Work out the finished part from the listing and answer in its coordinate system (mm). A direction names the side the tool comes from. Give positions to 0.01 mm unless a question says otherwise; leave off trailing zeros. Order: outer loops, then holes, each group sorted by start corner. A loop starts at its lowest first (then second) coordinate and runs counter-clockwise, first axis right, second up.
```python
from build123d import *

# Parameters (mm, degrees)
CYLINDER051_R       = 1.8
CYLINDER051_DEPTH   = 20
ARRAY001022_X_COUNT = 2
ARRAY001022_X_PITCH = 42
BOX022_W            = 122
BOX022_H            = 23
BOX022_DEPTH        = 1.4
BOX020_W            = 52
BOX020_H            = 22
BOX020_DEPTH        = 20
BOX019_W            = 62
BOX019_H            = 32
BOX019_DEPTH        = 5.2
FILLET010_R         = 0.7


with BuildPart() as obj1:
    # Cylinder051 → Cylinder051 (new body)
    with BuildSketch(Plane(origin=(10, 27, -5), x_dir=(1, 0, 0), z_dir=(0, 0, 1))):
        Circle(CYLINDER051_R)
    extrude(amount=CYLINDER051_DEPTH)

    # Array001022 X: obj1 ×2


with BuildPart() as obj1_1:
    add(obj1.part)
    with Locations(*[(i * ARRAY001022_X_PITCH, 0, 0) for i in range(1, ARRAY001022_X_COUNT)]):
        add(obj1.part)


with BuildPart() as obj2:
    # Box022 → Box022 (new body)
    with BuildSketch(Plane(origin=(-25, 0, 2), x_dir=(1, 0, 0), z_dir=(0, 0, 1))):
        with Locations((61, 11.5)):
            Rectangle(BOX022_W, BOX022_H)
    extrude(amount=BOX022_DEPTH)


with BuildPart() as obj3:
    # Box020 → Box020 (new body)
    with BuildSketch(Plane(origin=(5, 0, -10), x_dir=(1, 0, 0), z_dir=(0, 0, 1))):
        with Locations((26, 11)):
            Rectangle(BOX020_W, BOX020_H)
    extrude(amount=BOX020_DEPTH)

    # Fusion033: union obj2
    add(obj2.part)


with BuildPart() as obj4:
    # Box019 → Box019 (new body)
    with BuildSketch(Plane.XY):
        with Locations((31, 16)):
            Rectangle(BOX019_W, BOX019_H)
    extrude(amount=BOX019_DEPTH)

    # Cut019: cut obj3
    add(obj3.part, mode=Mode.SUBTRACT)

    # Fillet010
    fillet010_edges = [obj4.edges().sort_by_distance(p)[0] for p in [
        (0, 0, 1),
        (0, 0, 4.3),
        (0, 32, 2.6),
        (2.5, 0, 0),
        (5, 0, 1),
        (2.5, 0, 2),
        (59.5, 0, 2),
        (59.5, 0, 3.4),
        (2.5, 0, 3.4),
        (5, 0, 4.3),
        (2.5, 0, 5.2),
        (59.5, 0, 5.2),
        (62, 32, 2.6),
        (59.5, 0, 0),
        (62, 0, 1),
        (62, 0, 4.3),
        (57, 0, 1),
        (57, 0, 4.3),
    ]]
    fillet(fillet010_edges, radius=FILLET010_R)

    # Cut020: cut obj1
    add(obj1_1.part, mode=Mode.SUBTRACT)


solid = obj4.part
```
1. The part is cut by section C-C (x = 52). Write down the section's boundary in (y, z).
Findings below:
outline: (22, 0) - (25.2, 0) - (25.2, 5.2) - (22, 5.2) - (22, 3.4) - (23, 3.4) - (23, 2) - (22, 2) - close; (28.8, 0) - (32, 0) - (32, 5.2) - (28.8, 5.2) - close
2. Which of the six approach directions +Z, -Z, +X, -X, +Y, -Y give full straight-line access (tool end or side, diameter ignored) to faces 1 (the face through (57, 11, 1)), 2 (the face through (30.9, 22.6, 2)), 3 (the face through (9.766, 28.785, 2.564))?
Findings below:
face 1: +Z, -Z, -Y
face 2: +X, -X, -Y
face 3: +Z, -Z
3. The part is cut by section B-B (y = 21). Write down the section's boundary in (x, z), then the cut area to 3 significant figures.
Findings below:
outline: (0, 0) - (5, 0) - (5, 2) - (0, 2) - close; (0, 3.4) - (5, 3.4) - (5, 5.2) - (0, 5.2) - close; (57, 0) - (62, 0) - (62, 2) - (57, 2) - close; (57, 3.4) - (62, 3.4) - (62, 5.2) - (57, 5.2) - close
area: 38.0 mm2
4. Given P1, Ø11, axis at x = 20, y = 14.5, coming from the +Z side; P2, Ø0.5, axis at x = 41, z = 4.5, coming from the -Y side; P3, Ø0.7, axis at x = 18.5, z = 3, coming from the -Y side, each flat-ended and moving along its own axis, determine where each tip first touches the part or whether it passes through.
Findings below:
P1: passes through
P2: stops at y = 22
P3: stops at y = 23
5. The part is cut by section A-A (y = 27). Write down the section's boundary in (x, z).
Findings below:
outline: (0, 0) - (8.2, 0) - (8.2, 5.2) - (0, 5.2) - close; (11.8, 0) - (50.2, 0) - (50.2, 5.2) - (11.8, 5.2) - close; (53.8, 0) - (62, 0) - (62, 5.2) - (53.8, 5.2) - close
6. Straight lines are drawn through the part: probe 1 along X at (y, z) = (27, 2); probe 2 along X at (y, z) = (12, 3.8); probe 3 along Y at (x, z) = (10, 4.1). For each, find the intervals that lie inside material, in ascending order.
Findings below:
probe 1: x = 0 to 8.2, 11.8 to 50.2, 53.8 to 62
probe 2: x = 0 to 5, 57 to 62
probe 3: y = 22 to 25.2, 28.8 to 32
7. The part is cut by section D-D (x = 34.5). Write down the section's boundary in (y, z).
Findings below:
outline: (22, 0) - (32, 0) - (32, 5.2) - (22, 5.2) - (22, 3.4) - (23, 3.4) - (23, 2) - (22, 2) - close
8. The mould has two halves that part along Y. Classify faces 4 (the face through (62, 16, 1)), 5 (the face through (31, 22, 1)), 6 (the face through (51.766, 28.785, 2.564)): pulls with the +Y half, pulls with the -Y half, needs draft (parallel to the pull), parting line crosses it, or undercut.
Findings below:
face 4: needs draft
face 5: pulls with the -Y half
face 6: undercut
